Source: CAD feature listing. Evaluate the final solid. Frame: model axes, mm. A direction names the side the tool comes from. Give positions to 0.01 mm unless a question says otherwise; leave off trailing zeros. Order: outer loops, then holes, each group sorted by start corner. A loop starts at its lowest first (then second) coordinate and runs counter-clockwise, first axis right, second up. Notation, with made-up numbers: (17, -23.5) - (28, -23.5) arc R15 ccw to (28, -8.5) - close; hole circle Ø6 at (-12, 30.5). An arc over 180 degrees is marked (long way). Write each question's results on one line, items separated by ' | '. Start each with the question number.
Item 1: Section B-B on y = 21. Output: boundary loops of the cut face in (x, z), and give its area (3 significant figures).
Item 2: Set-up query: faces 1 (the flat face through (0, 0, 1.2)), 2 (the flat face through (-16, -10.8, 6)). Return all of +Z, -Z, +X, -X, +Y, -Y with unobstructed straight access to the full face (end or side cutting, diameter ignored); none if empty.
Item 3: Section A-A on x = 9. Output: boundary loops of the cut face in (y, z), and give its area (3 significant figures).
Item 4: Section D-D on z = 3.75. State how many separate pieces and enclosed holes the cut face has, and give its area (3 significant figures).
Item 5: Mould query, pull axis Y, two halves, no side actions, for faces 3 (the flat face through (0, -26.2, 10)), 4 (the flat face through (-15.59, -6.28, 9.05)), 5 (the flat face through (16, 8.7, 14)). Classes: released by +Y, released by -Y, zero draft, split by the parting line, or undercut.
Item 6: Contact query for a flat-ended pin moving along its axis: pin 1 Ø12 at (x, y) = (1, 8.5) entering from +Z. Output: stop coordinate, or through.
Item 7: Line query: line 1 along Y through (x, z) = (-14.5, 2); line 2 along X through (y, z) = (-21, 7.25); line 3 along Z through (x, y) = (-2.5, 0.5). Output: solid intervals per line, ascending.
Item 8: Section C-C on y = -23. Output: boundary loops of the cut face in (x, z).
```python
from build123d import *

# Parameters (mm, degrees)
SKETCH1_W           = 32.4
SKETCH1_H           = 52.4
BOSS_EXTRUDE1_DEPTH = 20
SHELL1_T            = -1.2
CUT_EXTRUDE1_DEPTH  = 47.219043694


with BuildPart() as part:
    # Sketch1 → Boss-Extrude1 (new body)
    with BuildSketch(Plane.XY):
        Rectangle(SKETCH1_W, SKETCH1_H)
    extrude(amount=BOSS_EXTRUDE1_DEPTH)

    # Shell1
    shell1_openings = [part.faces().sort_by_distance(p)[0] for p in [
        (0, 0, 20),
    ]]
    offset(amount=SHELL1_T, openings=shell1_openings, kind=Kind.INTERSECTION)

    # Sketch2 → Cut-Extrude1 (cut, through all)
    with BuildSketch(Plane(origin=(16.2, 0, 0), x_dir=(0, 0, -1), z_dir=(1, 0, 0))):
        Polygon((-3, 19.2), (-4.732050808, 22.2), (-8.196152423, 22.2), (-9.92820323, 19.2), (-8.196152423, 16.2), (-4.732050808, 16.2), align=None)
        Polygon((-3, 10.2), (-4.732050808, 13.2), (-8.196152423, 13.2), (-9.92820323, 10.2), (-8.196152423, 7.2), (-4.732050808, 7.2), align=None)
        Polygon((-10.794228634, 14.7), (-12.526279442, 17.7), (-15.990381057, 17.7), (-17.722431864, 14.7), (-15.990381057, 11.7), (-12.526279442, 11.7), align=None)
        Polygon((-3, 1.2), (-4.732050808, 4.2), (-8.196152423, 4.2), (-9.92820323, 1.2), (-8.196152423, -1.8), (-4.732050808, -1.8), align=None)
        Polygon((-3, -7.8), (-4.732050808, -4.8), (-8.196152423, -4.8), (-9.92820323, -7.8), (-8.196152423, -10.8), (-4.732050808, -10.8), align=None)
        Polygon((-3, -16.8), (-4.732050808, -13.8), (-8.196152423, -13.8), (-9.92820323, -16.8), (-8.196152423, -19.8), (-4.732050808, -19.8), align=None)
        Polygon((-10.794228634, 5.7), (-12.526279442, 8.7), (-15.990381057, 8.7), (-17.722431864, 5.7), (-15.990381057, 2.7), (-12.526279442, 2.7), align=None)
        Polygon((-10.794228634, -3.3), (-12.526279442, -0.3), (-15.990381057, -0.3), (-17.722431864, -3.3), (-15.990381057, -6.3), (-12.526279442, -6.3), align=None)
        Polygon((-10.794228634, -12.3), (-12.526279442, -9.3), (-15.990381057, -9.3), (-17.722431864, -12.3), (-15.990381057, -15.3), (-12.526279442, -15.3), align=None)
    extrude(amount=-CUT_EXTRUDE1_DEPTH, mode=Mode.SUBTRACT)


solid = part.part
```
Evaluation:
1) outline: (-16.2, 0) - (16.2, 0) - (16.2, 4.04) - (15, 4.04) - (15, 1.2) - (-15, 1.2) - (-15, 4.04) - (-16.2, 4.04) - close; (-16.2, 8.89) - (-15, 8.89) - (-15, 20) - (-16.2, 20) - close; (15, 8.89) - (16.2, 8.89) - (16.2, 20) - (15, 20) - close | area: 72.4 mm^2
2) face 1: +Z | face 2: +X, -X
3) outline: (-26.2, 0) - (26.2, 0) - (26.2, 20) - (25, 20) - (25, 1.2) - (-25, 1.2) - (-25, 20) - (-26.2, 20) - close | area: 108 mm^2
4) separate pieces: 10 | enclosed holes: 0 | area: 167 mm^2
5) face 3: released by -Y | face 4: undercut | face 5: undercut
6) pin 1: stops at z = 1.2
7) line 1: y = -26.2 to -25, 25 to 26.2 | line 2: x = -16.2 to -15, 15 to 16.2 | line 3: z = 0 to 1.2
8) outline: (-16.2, 0) - (16.2, 0) - (16.2, 20) - (15, 20) - (15, 1.2) - (-15, 1.2) - (-15, 20) - (-16.2, 20) - close
